from build123d import *

# Parameters (mm, degrees)
SKETCH2_W           = 88.9
SKETCH2_H           = 3.2004
BOSS_EXTRUDE1_DEPTH = 210.82
SKETCH3_R           = 1.1303
SKETCH3_R_2         = 5.08
CUT_EXTRUDE1_DEPTH  = 216.82004684
FILLET2_R           = 2.54


with BuildPart() as part:
    # Sketch2 → Boss-Extrude1 (new body)
    with BuildSketch(Plane.XY):
        with Locations((-1.625781684, -22.993244248)):
            Rectangle(SKETCH2_W, SKETCH2_H)
    extrude(amount=BOSS_EXTRUDE1_DEPTH)

    # Sketch3 → Cut-Extrude1 (cut, through all)
    with BuildSketch(Plane(origin=(0, -21.393044248, 0), x_dir=(-1, 0, 0), z_dir=(0, 1, 0))):
        with Locations(Location((14.833781684, 208.28, 0), (0, 0, 90))):
            Circle(SKETCH3_R)
        with Locations(Location((-11.683818316, 208.28, 0), (0, 0, 90))):
            Circle(SKETCH3_R)
        with Locations(Location((-7.619818316, 202.518755316, 0), (0, 0, 90))):
            Circle(SKETCH3_R_2)
        with Locations(Location((-33.478453416, 206.502, 0), (0, 0, 90))):
            Circle(SKETCH3_R)
        with Locations(Location((36.730016784, 206.502, 0), (0, 0, 90))):
            Circle(SKETCH3_R)
        with Locations(Location((-33.478453416, 4.318, 0), (0, 0, 90))):
            Circle(SKETCH3_R)
        with Locations(Location((36.730016784, 4.318, 0), (0, 0, 90))):
            Circle(SKETCH3_R)
        with Locations(Location((-18.450986138, 32.12110162, 0), (0, 0, 90))):
            Circle(SKETCH3_R)
        with Locations(Location((-18.450986138, 90.12110162, 0), (0, 0, 90))):
            Circle(SKETCH3_R)
        with Locations(Location((30.549013862, 90.12110162, 0), (0, 0, 90))):
            Circle(SKETCH3_R)
        with Locations(Location((30.549013862, 32.12110162, 0), (0, 0, 90))):
            Circle(SKETCH3_R)
        with Locations(Location((-21.181379204, 173.304632562, 0), (0, 0, 90))):
            Circle(SKETCH3_R)
        with Locations(Location((-36.421379204, 122.504632562, 0), (0, 0, 90))):
            Circle(SKETCH3_R)
        with Locations(Location((6.758620796, 173.304632562, 0), (0, 0, 90))):
            Circle(SKETCH3_R)
        with Locations(Location((11.838620796, 121.234632562, 0), (0, 0, 90))):
            Circle(SKETCH3_R)
        with Locations((81.579081393, -113.266782514)):
            Circle(SKETCH3_R)
        with Locations((66.769810529, -163.717742064)):
            Circle(SKETCH3_R)
        with Locations((108.318194793, -113.266782514)):
            Circle(SKETCH3_R)
        with Locations((97.604440284, -108.476314785)):
            Circle(SKETCH3_R)
        with Locations((82.79516942, -158.927274335)):
            Circle(SKETCH3_R)
        with Locations((124.343553684, -108.476314785)):
            Circle(SKETCH3_R)
        with Locations((112.789811005, -158.927274335)):
            Circle(SKETCH3_R)
        with BuildLine():
            Line((35.32929924, 12.595958552), (35.32929924, 133.302587666))
            ThreePointArc((35.32929924, 133.302587666), (38.50429924, 136.477587666), (41.67929924, 133.302587666))
            Line((41.67929924, 133.302587666), (41.67929924, 12.595958552))
            ThreePointArc((41.67929924, 12.595958552), (38.50429924, 9.420958552), (35.32929924, 12.595958552))
        make_face()
        with BuildLine():
            Line((-32.077737936, 12.595958552), (-32.077737936, 90.122587598))
            ThreePointArc((-32.077737936, 90.122587598), (-35.252737936, 93.297587598), (-38.427737936, 90.122587598))
            Line((-38.427737936, 90.122587598), (-38.427737936, 12.595958552))
            ThreePointArc((-38.427737936, 12.595958552), (-35.252737936, 9.420958552), (-32.077737936, 12.595958552))
        make_face()
    extrude(amount=-CUT_EXTRUDE1_DEPTH, mode=Mode.SUBTRACT)

    # Fillet2
    fillet2_edges = [part.edges().sort_by_distance(p)[0] for p in [
        (42.824218316, -22.993244248, 210.82),
        (-46.075781684, -22.993244248, 210.82),
        (42.824218316, -22.993244248, 0),
        (-46.075781684, -22.993244248, 0),
    ]]
    fillet(fillet2_edges, radius=FILLET2_R)


solid = part.part
Part model, mm, in its own coordinate system. Give positions to 0.01 mm unless a question says otherwise; leave off trailing zeros. Loops run counter-clockwise (first coordinate to the right, second up) from the corner with the lowest first, then second, coordinate; pieces in that order, holes last. Notation, with made-up numbers: (30, 17.5) -> (71, 17.5) arc R22 ccw to (71, 40.5) -> close; hole circle Ø11 at (71.25, 24). An arc over 180 degrees is marked (long way). Write each question's results on one line, items separated by ' | '. Start each with the question number.
Q1. Band-saw the part on B-B on z = 118. List the corners of the cut face in (x, y).
Q2. Pull direction Z, two halves, no side cores. Call faces 1 (the face through (5.67, -22.97, 207.21)), 2 (the face through (-2, -24.593, 104)): +Z half, -Z half, draft (parallel to the pull), parting line (faces both ways), or undercut.
Q3. Band-saw the part on A-A on z = 47. List the corners of the cut face in (x, y), plus the area to 3 significant figures.
Q4. Wall check: L1, parallel to X at y = -22.3, z = 51.5; L2, parallel to X at y = -23, z = 208.28; L3, parallel to Z at x = 21, y = -22.7. Give the ranges that are in metal, low to high.
Q5. Band-saw the part on C-C on y = -23.4. Count the separate pieces of the cut face and the enclosed holes in it, plus the area to 3 significant figures.
Q6. Pin check, flat tips, straight feed: P1, Ø1.4, axis at x = -14.83, z = 208.28, coming from the +Y side; P2, Ø11.5, axis at x = 7.62, z = 202.52, coming from the +Y side. Stop position of each tip, or through.
Results are:
1) outline: (-46.08, -24.59) -> (-41.68, -24.59) -> (-41.68, -21.39) -> (-46.08, -21.39) -> close; (-35.33, -24.59) -> (42.82, -24.59) -> (42.82, -21.39) -> (-35.33, -21.39) -> close
2) face 1: undercut | face 2: draft
3) outline: (-46.08, -24.59) -> (-41.68, -24.59) -> (-41.68, -21.39) -> (-46.08, -21.39) -> close; (-35.33, -24.59) -> (32.08, -24.59) -> (32.08, -21.39) -> (-35.33, -21.39) -> close; (38.43, -24.59) -> (42.82, -24.59) -> (42.82, -21.39) -> (38.43, -21.39) -> close | area: 244 mm²
4) L1: x = -46.08 to -41.68, -35.33 to 32.08, 38.43 to 42.82 | L2: x = -46.08 to -15.96, -13.7 to 10.55, 12.81 to 42.82 | L3: z = 0 to 172.19, 174.42 to 210.82
5) separate pieces: 1 | enclosed holes: 17 | area: 17,300 mm²
6) P1: passes through | P2: stops at y = -21.39
